Model file for the job. Use its own axes, mm. A direction names the side the tool comes from. Give positions to 0.01 mm unless a question says otherwise; leave off trailing zeros. Order: outer loops, then holes, each group sorted by start corner. A loop starts at its lowest first (then second) coordinate and runs counter-clockwise, first axis right, second up. Notation, with made-up numbers: (15.25, 29) - (33.25, 29) arc R19 ccw to (33.25, 34) - close; hole circle Ø9 at (-17.75, 29.5). An arc over 180 degrees is marked (long way). Use CSV: the item, a comma, the result in double quotes. Start each with the question number.
(1) Tool access for faces 1 (the cylindrical face through (97.64, 80.61, -50.89)), 2 (the cylindrical face through (113.14, 101.27, 54.67)), 3 (the cylindrical face through (17.19, 2.03, 34.75)): list every direction of +Z, -Z, +X, -X, +Y, -Y with a clear straight run to the whole face (end or side of a thin tool).
(2) Pull direction X, two halves, no side cores. Call faces 4 (the flat face through (169, 4, 47)), 5 (the cylindrical face through (7.7, 1.97, 38.68)), 6 (the flat face through (133, 4, -53)), 7 (the flat face through (55, 159, -24)): +X half, -X half, draft (parallel to the pull), parting line (faces both ways), or undercut.
(3) Band-saw the part on C-C, the plane y = 145. Give the cut face in (x, z).
(4) Probe L1, parallel to Z at x = 101, y = 1; L2, parallel to X at y = 1.2, z = 0; L3, parallel to Z at x = 101, y = 52. List the from-to ranges inside material, lowest first.
(5) Drop flat-ended pins along their axis: pin 1 Ø6 at (y, z) = (25, 35.5) entering from -X; pin 2 Ø10 at (x, y) = (93.5, 36.5) entering from +Z; pin 3 Ø8 at (y, z) = (40.5, 53) entering from +X. Give the stop position or say it passes through.
from build123d import *

# Parameters (mm, degrees)
CUT_EXTRUDE1_REACH = 161
SKETCH2_R          = 51


with BuildPart() as part:
    # Sketch1 → Revolve1 (revolve)
    with BuildSketch(Plane.XY):
        Polygon((50, 159), (0, 159), (0, 154), (45, 154), (45, 50), (0, 4), (0, 0), (10.27, 0), (10.27, 4), (19.87, 4), (19.87, 0), (30.14, 0), (30.14, 4), (39.74, 4), (39.74, 0), (50, 0), (101, 0), (101, 4), (50, 4), align=None)
    revolve(axis=Axis((101, 4, 0), (0, -1, 0)))

    # Sketch2 → Cut-Extrude1 (cut, up to next)
    with BuildSketch(Plane.XZ, mode=Mode.PRIVATE) as cut_extrude1_sk1:
        with Locations((101, 0)):
            Circle(SKETCH2_R)
    cut_extrude1_tool1 = extrude(cut_extrude1_sk1.sketch, amount=-CUT_EXTRUDE1_REACH, mode=Mode.PRIVATE) & part.part
    add(cut_extrude1_tool1.solids().sort_by_distance((101, 0, 0))[0], mode=Mode.SUBTRACT)


solid = part.part
Answer block:
1,face 1,"+Y, -Y"
1,face 2,"none"
1,face 3,"-Y"
2,face 4,"undercut"
2,face 5,"parting line"
2,face 6,"undercut"
2,face 7,"draft"
3,outline,"circle Ø112 at (101, 0); hole circle Ø102 at (101, 0)"
4,L1,"z = -101 to -90.73, -81.13 to -70.86, -61.26 to -51, 51 to 61.26, 70.86 to 81.13, 90.73 to 101"
4,L2,"x = 0 to 10.27, 19.87 to 30.14, 39.74 to 50, 152 to 162.26, 171.86 to 182.13, 191.73 to 202"
4,L3,"z = -56 to -51, 51 to 56"
5,pin 1,"stops at x = 25.26"
5,pin 2,"stops at z = 73.74"
5,pin 3,"stops at x = 147.06"
